Read the model definition and answer for the solid it produces. Units are mm, in the model's axes. Give positions to 0.01 mm unless a question says otherwise; leave off trailing zeros. Write each question's results on one line, items separated by ' | '. Start each with the question number.
Item 1: Section A-A on z = 2.5 is taken. State how many separate pieces and enclosed holes the cut face has, and give its area (3 significant figures).
Item 2: Each of these flat-tipped pins is pushed along its axis until it touches: P1, Ø3, axis at y = 37, z = 3.5, coming from the +X side; P2, Ø1.7, axis at x = -95.5, z = 3.5, coming from the +Y side; P3, Ø3, axis at x = -203.5, y = 24.88, coming from the -Z side; P4, Ø3, axis at y = 37.5, z = 3, coming from the -X side. Where does it stop, or does it pass through?
Item 3: Find the intervals of material crossed by line 1 (Y direction, x = -290.53, z = 1.35); line 2 (X direction, y = -22.5, z = 0.8); line 3 (Y direction, x = -196.5, z = 2.7), in increasing order.
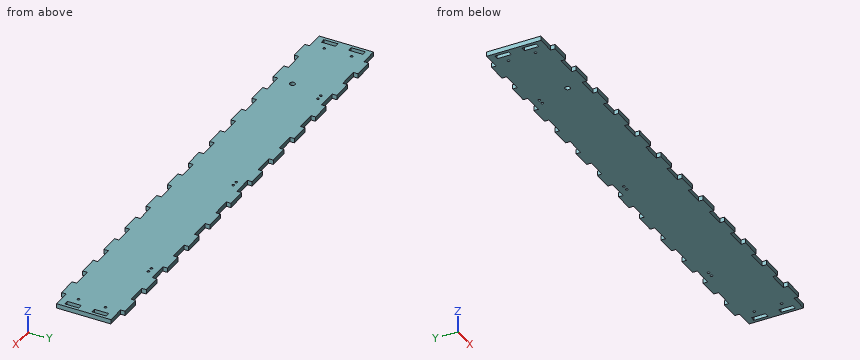
```python
from build123d import *

# Parameters (mm, degrees)
SKETCH1_R           = 3.3
SKETCH1_R_2         = 1.55
SKETCH1_W           = 5.85
SKETCH1_H           = 18
BOSS_EXTRUDE1_DEPTH = 5.8


with BuildPart() as part:
    # Sketch1 → Boss-Extrude1 (new body)
    with BuildSketch(Plane.XY):
        Polygon((-237.5, 34.5), (-237.5, 40.3), (-212.6, 40.3), (-212.6, 34.5), (-187.5, 34.5), (-187.5, 40.3), (-162.6, 40.3), (-162.6, 34.5), (-137.5, 34.5), (-137.5, 40.3), (-112.6, 40.3), (-112.6, 34.5), (-87.5, 34.5), (-87.5, 40.3), (-62.6, 40.3), (-62.6, 34.5), (-37.5, 34.5), (-37.5, 40.3), (-12.6, 40.3), (-12.6, 34.5), (12.5, 34.5), (12.5, 40.3), (37.4, 40.3), (37.4, 34.5), (62.5, 34.5), (62.5, 40.3), (87.4, 40.3), (87.4, 34.5), (112.5, 34.5), (112.5, 40.3), (137.4, 40.3), (137.4, 34.5), (162.5, 34.5), (162.5, 40.3), (187.4, 40.3), (187.4, 34.5), (212.5, 34.5), (212.5, 40.3), (237.4, 40.3), (237.4, 34.5), (262.5, 34.5), (262.5, 40.3), (287.4, 40.3), (287.4, 34.5), (310, 34.5), (310, -34.5), (287.4, -34.5), (287.4, -40.3), (262.5, -40.3), (262.5, -34.5), (237.4, -34.5), (237.4, -40.3), (212.5, -40.3), (212.5, -34.5), (187.4, -34.5), (187.4, -40.3), (162.5, -40.3), (162.5, -34.5), (137.4, -34.5), (137.4, -40.3), (112.5, -40.3), (112.5, -34.5), (87.4, -34.5), (87.4, -40.3), (62.5, -40.3), (62.5, -34.5), (37.4, -34.5), (37.4, -40.3), (12.5, -40.3), (12.5, -34.5), (-12.6, -34.5), (-12.6, -40.3), (-37.5, -40.3), (-37.5, -34.5), (-62.6, -34.5), (-62.6, -40.3), (-87.5, -40.3), (-87.5, -34.5), (-112.6, -34.5), (-112.6, -40.3), (-137.5, -40.3), (-137.5, -34.5), (-162.6, -34.5), (-162.6, -40.3), (-187.5, -40.3), (-187.5, -34.5), (-212.6, -34.5), (-212.6, -40.3), (-237.5, -40.3), (-237.5, -34.5), (-262.6, -34.5), (-262.6, -40.3), (-287.5, -40.3), (-287.5, -34.5), (-310, -34.5), (-310, 34.5), (-287.5, 34.5), (-287.5, 40.3), (-262.6, 40.3), (-262.6, 34.5), align=None)
        with Locations((-210, -14.5)):
            Circle(SKETCH1_R, mode=Mode.SUBTRACT)
        with Locations((-290.53, 17.25)):
            Circle(SKETCH1_R_2, mode=Mode.SUBTRACT)
        with Locations(Location((-290.53, -17.25, 0), (0, 0, 180))):
            Circle(SKETCH1_R_2, mode=Mode.SUBTRACT)
        with Locations((290.53, -17.25)):
            Circle(SKETCH1_R_2, mode=Mode.SUBTRACT)
        with Locations(Location((290.53, 17.25, 0), (0, 0, 180))):
            Circle(SKETCH1_R_2, mode=Mode.SUBTRACT)
        with Locations((3.5, 24.88)):
            Circle(SKETCH1_R_2, mode=Mode.SUBTRACT)
        with Locations(Location((-3.5, 24.88, 0), (0, 0, 180))):
            Circle(SKETCH1_R_2, mode=Mode.SUBTRACT)
        with Locations(Location((196.5, 24.88, 0), (0, 0, 180))):
            Circle(SKETCH1_R_2, mode=Mode.SUBTRACT)
        with Locations((203.5, 24.88)):
            Circle(SKETCH1_R_2, mode=Mode.SUBTRACT)
        with Locations((-196.5, 24.88)):
            Circle(SKETCH1_R_2, mode=Mode.SUBTRACT)
        with Locations(Location((-203.5, 24.88, 0), (0, 0, 180))):
            Circle(SKETCH1_R_2, mode=Mode.SUBTRACT)
        with Locations((303.075, 17.25)):
            Rectangle(SKETCH1_W, SKETCH1_H, mode=Mode.SUBTRACT)
        with Locations((303.075, -17.25)):
            Rectangle(SKETCH1_W, SKETCH1_H, mode=Mode.SUBTRACT)
        with Locations((-303.075, -17.25)):
            Rectangle(SKETCH1_W, SKETCH1_H, mode=Mode.SUBTRACT)
        with Locations((-303.075, 17.25)):
            Rectangle(SKETCH1_W, SKETCH1_H, mode=Mode.SUBTRACT)
    extrude(amount=BOSS_EXTRUDE1_DEPTH)


solid = part.part
```
Findings:
1) separate pieces: 1 | enclosed holes: 15 | area: 45,700 mm2
2) P1: x = 287.4 | P2: y = 34.5 | P3: through | P4: x = -287.5
3) line 1: -34.5 to -18.8, -15.7 to 15.7, 18.8 to 34.5 | line 2: -310 to -306, -300.15 to 300.15, 306 to 310 | line 3: -34.5 to 23.33, 26.43 to 34.5
